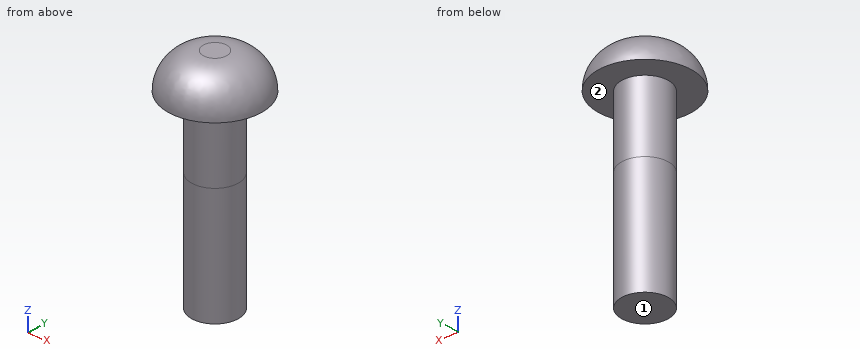
Autodesk Inventor part; units mm, degrees
ref_plane "YZ Plane" through (0, 0, 0) normal (1, 0, 0) x (0, 1, 0)
ref_plane "XZ Plane" through (0, 0, 0) normal (0, 1, 0) x (-1, 0, 0)
ref_plane "XY Plane" through (0, 0, 0) normal (0, 0, 1) x (1, 0, 0)
sketch "スケッチ1" plane through (0, 0, 0) normal (0, 0, 1) x (1, 0, 0)
  circle A0 centre (0, 0) radius 2
  dimension "d0" = 4
extrude "押し出し1" add sketch "スケッチ1" along normal blind 6
sketch "スケッチ2" plane through (0, 0, 6) normal (0, 0, 1) x (1, 0, 0)
  circle A0 centre (0, 0) radius 2
  circle A1 centre (0, 0) radius 4
  dimension "d3" = 8
extrude "押し出し2" add sketch "スケッチ2" along normal blind 3 contours A0 | A1
fillet "フィレット1" radius 3 1 edges at (-4, 0, 9)
thread "ねじ1"
sketch "スケッチ3" plane through (0, 0, 0) normal (0, 0, -1) x (-1, 0, 0)
  circle A0 centre (0, 0) radius 2
extrude "押し出し3" add sketch "スケッチ3" along normal blind 10
properties part number "SB　M4 16mm なべネジ" material "Stainless Steel, 440C"
Geometry: final body of the model. Coordinates: model frame, mm. Face numbers are marked on the shaded views. A direction names the side the tool comes from. Give positions to 0.01 mm unless a question says otherwise; leave off trailing zeros. Loops run counter-clockwise (first coordinate to the right, second up) from the corner with the lowest first, then second, coordinate; pieces in that order, holes last. Notation, with made-up numbers: (64, 73.25) -> (89, 73.25) arc R29 ccw to (89, 95.25) -> close; hole circle Ø2 at (11, 4). An arc over 180 degrees is marked (long way). Return JSON: item names as keys, results as strings.
Item 1: Pin query (flat end, axial travel): P1, Ø2, axis at y = 1, z = 4.5, coming from the +X side; P2, Ø1.5, axis at x = -1, y = -2.5, coming from the -Z side; P3, Ø3, axis at y = -2, z = 0, coming from the -X side; P4, Ø1, axis at y = 2, z = -8, coming from the +X side. Return the tip coordinate at first contact, or that it passes through.
Filled in:
{"P1": "x = 2", "P2": "z = -10", "P3": "x = -1.94", "P4": "x = 1.32"}
Item 2: Access query for the marked faces 1 and 2. Directions: +Z, -Z, +X, -X, +Y, -Y. A direction counts if a zero-diameter tool reaches every point of the face in a straight line with its end or side. Return the directions, or none.
Filled in:
{"face 1": "-Z, +X, -X, +Y, -Y", "face 2": "-Z"}
Item 3: Line query: line 1 (X direction, y = 0, z = 4.25); line 2 (Z direction, x = -1.5, y = 2.5); line 3 (Y direction, x = 1.25, z = -8.75). Output: solid intervals per line, ascending.
Filled in:
{"line 1": "-2 to 2", "line 2": "6 to 8.31", "line 3": "-1.56 to 1.56"}
Item 4: Section A-A, the plane z = -1. Output: boundary loops of the cut face in (x, y).
Filled in:
{"outline": "circle Ø4 at (0, 0)"}
